Here's the drawing with two shaded views (mm, measured from the low corner). I have some questions. A direction names the side the tool comes from. Round coordinates to 2 decimals unless told otherwise and drop trailing zeros. Loops run counter-clockwise (first coordinate to the right, second up) from the corner with the lowest first, then second, coordinate; pieces in that order, holes last.
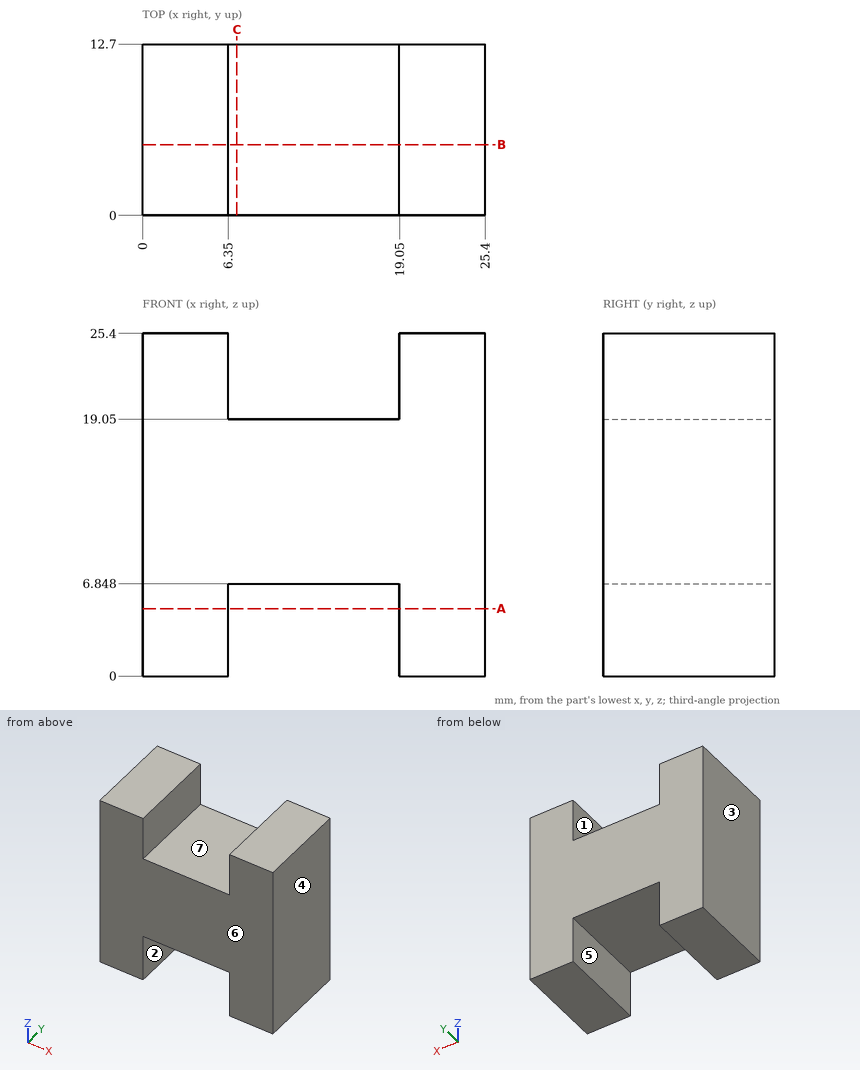
Item 1: If we section it at A-A, the plane z = 5: Please give me the cut outline in (x, y).
Results list:
outline: (0, 0) - (6.35, 0) - (6.35, 12.7) - (0, 12.7) - close; (19.05, 0) - (25.4, 0) - (25.4, 12.7) - (19.05, 12.7) - close
Item 2: If I drill on line 1 along X through (y, z) = (11, 1.75); line 2 along Z through (x, y) = (18.5, 6.5), over which ranges is the centre line in solid material (lowest first)?
Results list:
line 1: x = 0 to 6.35, 19.05 to 25.4
line 2: z = 6.85 to 19.05
Item 3: We'd pull the mould along X, two halves only. Please class the marked faces 1, 2, 3 and 4: released by +X, released by -X, zero draft, split by the parting line, or undercut.
Results list:
face 1: undercut
face 2: undercut
face 3: released by -X
face 4: released by +X
Item 4: For the marked faces 5, 6 and 7, which set-ups out of +Z, -Z, +X, -X, +Y, -Y let a thin tool reach every point of the face, with its end or its side?
Results list:
face 5: -Z, +Y, -Y
face 6: +Z, -Z, +X, -X, -Y
face 7: +Z, +Y, -Y
Item 5: If we section it at B-B, the plane y = 5.25: Please give me the cut outline in (x, z), then the cut area to 3 significant figures.
Results list:
outline: (0, 0) - (6.35, 0) - (6.35, 6.85) - (19.05, 6.85) - (19.05, 0) - (25.4, 0) - (25.4, 25.4) - (19.05, 25.4) - (19.05, 19.05) - (6.35, 19.05) - (6.35, 25.4) - (0, 25.4) - close
area: 478 mm2
Item 6: If we section it at C-C, the plane x = 7: Please give me the cut outline in (y, z).
Results list:
outline: (0, 6.85) - (12.7, 6.85) - (12.7, 19.05) - (0, 19.05) - close
Item 7: Will this pin go through, and if not, where does the flat tip stop? pin 1 (5 mm diameter, centred on x = 10, y = 4.5, fed in from +Z).
Results list:
pin 1: stops at z = 19.05
